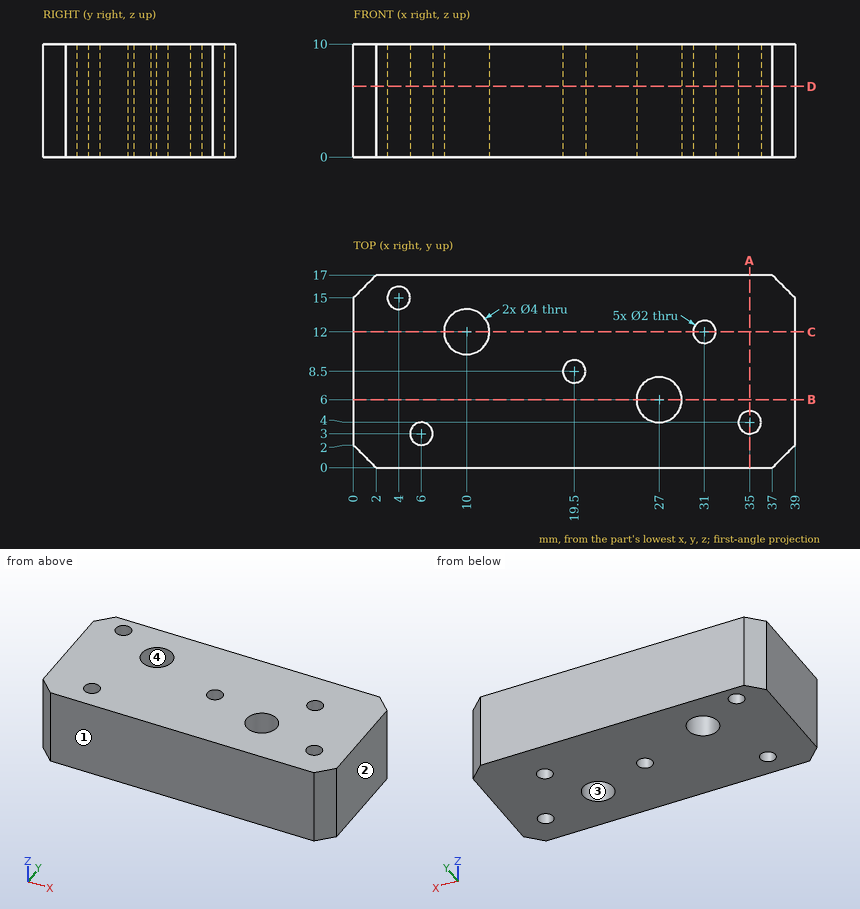
Design review of the part shown in the three views and the two pictorial views. Dimensions are in mm from the part's minimum x, y and z. Coordinates: 2 decimals unless noted, no trailing zeros. Loops run counter-clockwise (first coordinate to the right, second up) from the corner with the lowest first, then second, coordinate; pieces in that order, holes last. Notation, with made-up numbers: (-12, -39) - (18, -39) arc R14 ccw to (18, -33) - close; hole circle Ø2 at (47, -32). An arc over 180 degrees is marked (long way). Use a Markdown table: item, result. Add a question column.
Item 1: For line 1 (Y direction, x = 35, z = 3.5); line 2 (X direction, y = 3.5, z = 1.5); line 3 (X direction, y = 11.75, z = 1), list the stretches that pass through material, from the lowest coordinate up.
Item 2: We need section B-B (y = 6). Give the boundary of the cut face in (x, z), and give its area (3 significant figures).
Item 3: We need section A-A (x = 35). Give the boundary of the cut face in (y, z).
Item 4: Mouldability with a two-part tool opening along Y and no side actions: class the marked faces 1, 2, 3 and 4 as pulls with the +Y half, pulls with the -Y half, needs draft (parallel to the pull), parting line crosses it, or undercut.
Item 5: We need section D-D (z = 6.25). Give the boundary of the cut face in (x, y).
Item 6: We need section C-C (y = 12). Give the boundary of the cut face in (x, z), and give its area (3 significant figures).
Item 7: Insertion check: pin 1 Ø1.2 at (x, y) = (35, 4) entering from +Z. The pin has a flat end and moves straight along its axis. Give the tip position at first contact, or say it passes through.
Results list:
| question | item | result |
|---|---|---|
| 1 | line 1 | y = 0 to 3, 5 to 17 |
| 1 | line 2 | x = 0 to 5.13, 6.87 to 34.13, 35.87 to 39 |
| 1 | line 3 | x = 0 to 8.02, 11.98 to 30.03, 31.97 to 39 |
| 2 | outline | (0, 0) - (25, 0) - (25, 10) - (0, 10) - close; (29, 0) - (39, 0) - (39, 10) - (29, 10) - close |
| 2 | area | 350 mm^2 |
| 3 | outline | (0, 0) - (3, 0) - (3, 10) - (0, 10) - close; (5, 0) - (17, 0) - (17, 10) - (5, 10) - close |
| 4 | face 1 | pulls with the -Y half |
| 4 | face 2 | needs draft |
| 4 | face 3 | undercut |
| 4 | face 4 | undercut |
| 5 | outline | (0, 2) - (2, 0) - (37, 0) - (39, 2) - (39, 15) - (37, 17) - (2, 17) - (0, 15) - close; hole circle Ø2 at (4, 15); hole circle Ø2 at (6, 3); hole circle Ø4 at (10, 12); hole circle Ø2 at (19.5, 8.5); hole circle Ø4 at (27, 6); hole circle Ø2 at (31, 12); hole circle Ø2 at (35, 4) |
| 6 | outline | (0, 0) - (8, 0) - (8, 10) - (0, 10) - close; (12, 0) - (30, 0) - (30, 10) - (12, 10) - close; (32, 0) - (39, 0) - (39, 10) - (32, 10) - close |
| 6 | area | 330 mm^2 |
| 7 | pin 1 | passes through |
